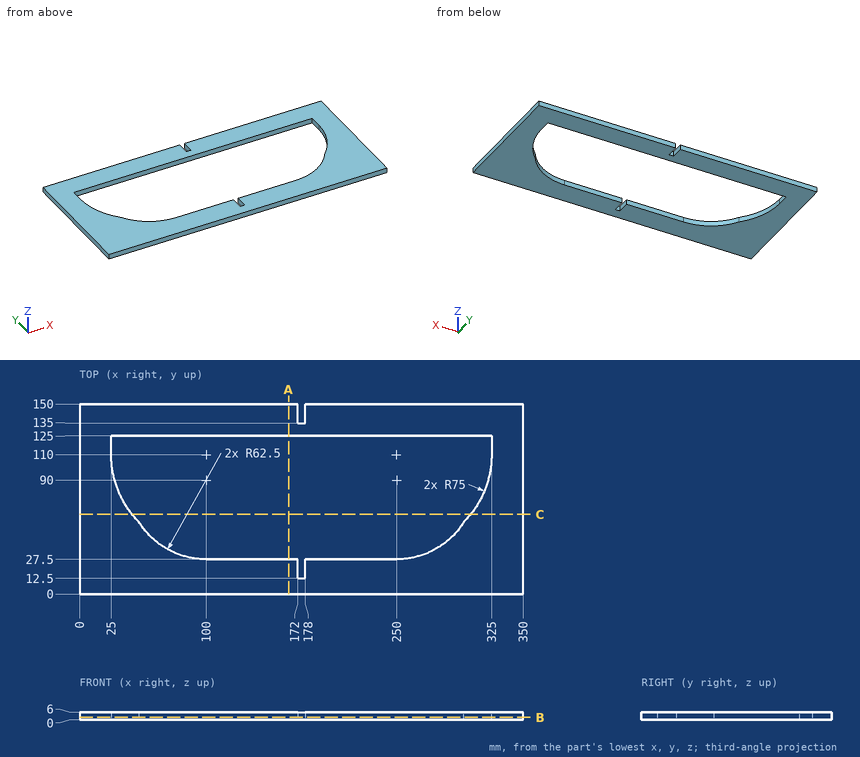
Design review of the part shown in the three views and the two pictorial views. Dimensions are in mm from the part's minimum x, y and z. Round coordinates to 2 decimals unless told otherwise and drop trailing zeros. Loops run counter-clockwise (first coordinate to the right, second up) from the corner with the lowest first, then second, coordinate; pieces in that order, holes last. Notation, with made-up numbers: (-23.75, 59) -> (-18.75, 59) arc R20 ccw to (-18.75, 88) -> close; hole circle Ø9 at (88.25, -10). An arc over 180 degrees is marked (long way). Answer as a JSON object with one key per item and string values. Group by question number.
1) We need section B-B on z = 1.85. Write out the cut boundary in (x, y), then the cut area to 3 significant figures.
2) For line 1 (X direction, y = 112, z = 5.75); line 2 (X direction, y = 140.5, z = 5); line 3 (Y direction, x = 131, z = 2.65), list the stretches that pass through material, from the lowest coordinate up. Write a range as [from, to].
3) For pin 1 Ø1.8 at (x, z) = (175, 3) entering from +Y, flat-tipped, find the tip position at first contact; note if it passes through.
4) We need section C-C on y = 63. Write out the cut boundary in (x, z).
5) We need section A-A on x = 165. Write out the cut boundary in (y, z), then the cut area to 3 significant figures.
Result set:
{
 "1": {"outline": "(0, 0) -> (350, 0) -> (350, 150) -> (178, 150) -> (178, 135) -> (172, 135) -> (172, 150) -> (0, 150) -> close; hole (25, 110) arc R75 ccw to (46.9, 57.03) arc R62.5 ccw to (100, 27.5) -> (172, 27.5) -> (172, 12.5) -> (178, 12.5) -> (178, 27.5) -> (250, 27.5) arc R62.5 ccw to (303.1, 57.03) arc R75 ccw to (325, 110) -> (325, 125) -> (25, 125) -> close", "area": "26,000 mm²"},
 "2": {"line 1": "[0, 25], [325, 350]", "line 2": "[0, 172], [178, 350]", "line 3": "[0, 27.5], [125, 150]"},
 "3": {"pin 1": "y = 135"},
 "4": {"outline": "(0, 0) -> (41.55, 0) -> (41.55, 6) -> (0, 6) -> close; (308.45, 0) -> (350, 0) -> (350, 6) -> (308.45, 6) -> close"},
 "5": {"outline": "(0, 0) -> (27.5, 0) -> (27.5, 6) -> (0, 6) -> close; (125, 0) -> (150, 0) -> (150, 6) -> (125, 6) -> close", "area": "315 mm²"}
}
